Geometry check sheet. Reference: the model listing, model coordinates, mm. Give positions to 0.01 mm unless a question says otherwise; leave off trailing zeros. Order: outer loops, then holes, each group sorted by start corner. A loop starts at its lowest first (then second) coordinate and runs counter-clockwise, first axis right, second up. Notation, with made-up numbers: (-0.5, 29.25) - (39.5, 29.25) arc R32 ccw to (39.5, 63.25) - close; hole circle Ø3 at (40.5, 83). An arc over 180 degrees is marked (long way). Put each result on its own line as item: value. Start each with the question number.
```python
from build123d import *

# Parameters (mm, degrees)
CROQUIS1_W     = 530
CROQUIS1_H     = 530
EXTRUIR1_DEPTH = 3
CROQUIS3_R     = 79.5
EXTRUIR2_DEPTH = 375.77860131


with BuildPart() as part:
    # Croquis1 → Extruir1 (new body)
    with BuildSketch(Plane(origin=(0, 0, 0), x_dir=(0, -1, 0), z_dir=(1, 0, 0))):
        Rectangle(CROQUIS1_W, CROQUIS1_H)
    extrude(amount=EXTRUIR1_DEPTH)

    # Croquis3 → Extruir2 (cut, through all)
    with BuildSketch(Plane.ZY):
        Circle(CROQUIS3_R)
    extrude(amount=-EXTRUIR2_DEPTH, mode=Mode.SUBTRACT)


solid = part.part
```
Item 1: Cross-section at C-C (x = 2.3). Enter the section's corners in (y, z).
Item 2: Cross-section at A-A (y = 0). Enter the section's corners in (x, z).
Item 3: Release check for a two-part mould opening along Y. For faces 1 (the face through (1.479, 78.823, -10.349)), 2 (the face through (0, 63, -63)) record: +Y half, -Y half, draft (parallel to the pull), parting line (faces both ways), or undercut.
Item 4: Thickness scan on line 1 along Y through (x, z) = (0.7, 0); line 2 along Z through (x, y) = (1.45, -29); line 3 along Z through (x, y) = (1.7, -18). Record the ranges inside material, lowest first.
Recorded:
1. outline: (-265, -265) - (265, -265) - (265, 265) - (-265, 265) - close; hole circle Ø159 at (0, 0)
2. outline: (0, -265) - (3, -265) - (3, -79.5) - (0, -79.5) - close; (0, 79.5) - (3, 79.5) - (3, 265) - (0, 265) - close
3. face 1: undercut
3. face 2: draft
4. line 1: y = -265 to -79.5, 79.5 to 265
4. line 2: z = -265 to -74.02, 74.02 to 265
4. line 3: z = -265 to -77.44, 77.44 to 265
